Build history of the part. All positions in model axes, mm. Coordinates: 2 decimals unless noted, no trailing zeros. Write each loop counter-clockwise with the first axis right and the second up, starting at its lowest first coordinate (ties: lowest second). Pieces come first, ordered by that corner, then holes. Notation, with made-up numbers: M -15,-28 L -6,-28 A5 cw -6,-24 Z; hole C 70,44 d10. An arc over 180 degrees is marked long. Use CSV: the item, a comma, the result in double quotes. Start each with the question number.
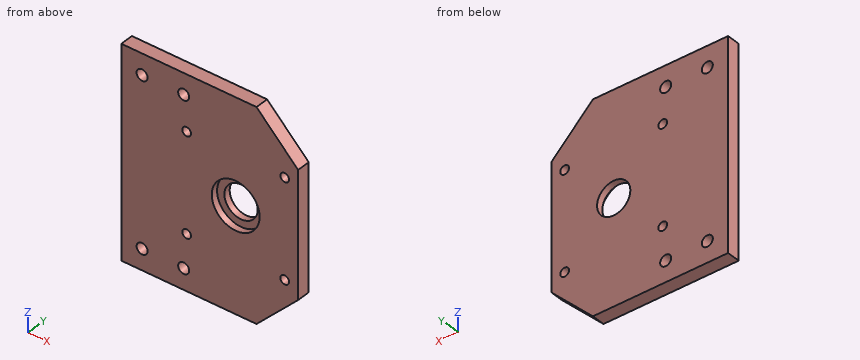
```python
from build123d import *

# Parameters (mm, degrees)
BOSS_EXTRUDE1_DEPTH   = 6.35
M5X0_8_TAPPED_HOLE1_D = 4.2
M5_CLEARANCE_HOLE1_D  = 5.3
SKETCH6_R             = 11.5
CUT_EXTRUDE1_DEPTH    = 3.175
SKETCH7_R             = 8
CUT_EXTRUDE2_DEPTH    = 10


with BuildPart() as part:
    # Sketch1 → Boss-Extrude1 (new body)
    with BuildSketch(Plane(origin=(0, 0, 0), x_dir=(1, 0, 0), z_dir=(0, 1, 0))):
        Polygon((0, 0), (65, 0), (85, -20), (85, -80), (65, -100), (0, -100), align=None)
    extrude(amount=BOSS_EXTRUDE1_DEPTH)

    # M5x0.8 Tapped Hole1 (through all)
    with Locations(Plane(origin=(0, 6.35, 0), x_dir=(1, 0, 0), z_dir=(0, 1, 0))):
        with Locations((78.57, -26.43), (31.43, -26.43), (31.43, -73.57), (78.57, -73.57)):
            Hole(M5X0_8_TAPPED_HOLE1_D / 2)

    # M5 Clearance Hole1 (through all)
    with Locations(Plane(origin=(0, 6.35, 0), x_dir=(1, 0, 0), z_dir=(0, 1, 0))):
        with Locations((10, -10), (30, -10), (10, -90), (30, -90)):
            Hole(M5_CLEARANCE_HOLE1_D / 2)

    # Sketch6 → Cut-Extrude1 (cut)
    with BuildSketch(Plane(origin=(0, 0, 0), x_dir=(1, 0, 0), z_dir=(0, 1, 0))):
        with Locations((55, -50)):
            Circle(SKETCH6_R)
    extrude(amount=CUT_EXTRUDE1_DEPTH, mode=Mode.SUBTRACT)

    # Sketch7 → Cut-Extrude2 (cut)
    with BuildSketch(Plane(origin=(0, 3.175, 0), x_dir=(-1, 0, 0), z_dir=(0, -1, 0))):
        with Locations((-55, -50)):
            Circle(SKETCH7_R)
    extrude(amount=-CUT_EXTRUDE2_DEPTH, mode=Mode.SUBTRACT)


solid = part.part
```
1. Slice it at D-D (z = 56.5). List the corners of the cut face in (x, y) (3 decimals), and give its area (3 significant figures).
2. Drill centre lines: line 1 along Z through (x, y) = (10, 3); line 2 along X through (y, z) = (4, 10); line 3 along X through (y, z) = (0.5, 28). Where is each one in solid material? Low to high. Write a range as from..to.
3. Flat gauge pins, fed straight in: pin 1 (3 mm diameter, centred on x = 10, z = 10, fed in from -Y); pin 2 (1.5 mm diameter, centred on x = 67.5, y = 4.5, fed in from -Z); pin 3 (18.5 mm diameter, centred on x = 55, z = 50, fed in from -Y) (3 decimals). Where does each tip first touch, or does it go through?
4. Slice it at A-A (z = 90). List the corners of the cut face in (x, y), and give its area (3 significant figures).
5. Slice it at C-C (x = 55). List the corners of the cut face in (y, z) (3 decimals), and give its area (3 significant figures).
6. Slice it at B-B (x = 10). List the corners of the cut face in (y, z).
Established:
1,outline,"M 0,0 L 45.513,0 L 45.513,3.175 L 50.336,3.175 L 50.336,6.35 L 0,6.35 Z; M 59.664,3.175 L 64.487,3.175 L 64.487,0 L 85,0 L 85,6.35 L 59.664,6.35 Z"
1,area,"450 mm2"
2,line 1,"z = 0..7.35, 12.65..87.35, 92.65..100"
2,line 2,"x = 0..7.35, 12.65..27.35, 32.65..75"
2,line 3,"x = 0..30.04, 32.82..77.18, 79.96..85"
3,pin 1,"passes through"
3,pin 2,"stops at z = 1.75"
3,pin 3,"stops at y = 3.175"
4,outline,"M 0,0 L 7.35,0 L 7.35,6.35 L 0,6.35 Z; M 12.65,0 L 27.35,0 L 27.35,6.35 L 12.65,6.35 Z; M 32.65,0 L 75,0 L 75,6.35 L 32.65,6.35 Z"
4,area,"409 mm2"
5,outline,"M 0,0 L 6.35,0 L 6.35,42 L 3.175,42 L 3.175,38.5 L 0,38.5 Z; M 0,61.5 L 3.175,61.5 L 3.175,58 L 6.35,58 L 6.35,100 L 0,100 Z"
5,area,"511 mm2"
6,outline,"M 0,0 L 6.35,0 L 6.35,7.35 L 0,7.35 Z; M 0,12.65 L 6.35,12.65 L 6.35,87.35 L 0,87.35 Z; M 0,92.65 L 6.35,92.65 L 6.35,100 L 0,100 Z"
